Read the model definition and answer for the solid it produces. Units are mm, in the model's axes. A direction names the side the tool comes from. Round coordinates to 2 decimals unless told otherwise and drop trailing zeros. Write each loop counter-clockwise with the first axis right and the second up, starting at its lowest first coordinate (ties: lowest second). Pieces come first, ordered by that corner, then holes. Notation, with made-up numbers: (78.5, 85.25) - (118.5, 85.25) arc R16 cw to (118.5, 104.25) - close; hole circle Ø5 at (86, 26). An arc over 180 degrees is marked (long way). Use one line per item in the form item = value. Start each with the question number.
1) For a pull along Y with two mould halves and no side action, classify faces 1 (the face through (-12, -8, -5)), 2 (the face through (0, -2.8, 9.3)), 3 (the face through (-0.61, 13, 4.09)) as released by +Y, released by -Y, zero draft, split by the parting line, or undercut.
2) Consider line 1 along X through (y, z) = (16, -9.5); line 2 along Z through (x, y) = (-6.5, 12); line 3 along Z through (x, y) = (-7, -17.5). Determine where each line is inside the solid, lowest interval first. Write a range as from..to.
3) For faces 4 (the face through (-2, 13, -13)), 5 (the face through (-6.206, 4.57, 7.167)), 6 (the face through (-11.47, -1.46, 11.12)), determine the directions among +Z, -Z, +X, -X, +Y, -Y from which every point of the face is accessible in a straight line to the end or side of a thin tool.
4) The part is cut by section B-B, the plane x = -8. Give the vertices of the cut face in (y, z), plus the area to 3 significant figures.
5) The part is cut by section A-A, the plane x = -10.25. Give the vertices of the cut face in (y, z).
6) Each of these flat-tipped pins is pushed along its axis until it touches: pin 1 (3 mm diameter, centred on x = -8, y = 12.5, fed in from -Z); pin 2 (15.5 mm diameter, centred on y = 0, z = 0, fed in from -X); pin 3 (2 mm diameter, centred on x = -2, z = -3.5, fed in from -Y); pin 4 (6 mm diameter, centred on x = -10, z = -9, fed in from +Y). Where does it stop, or does it pass through?
from build123d import *


with BuildPart() as part:
    # OutRacSke → OuterRace (revolve)
    with BuildSketch(Plane.XY):
        with BuildLine():
            Line((-2, 18.15674466), (-13, 15.704))
            Line((-13, 15.704), (-13, 19))
            ThreePointArc((-13, 19), (-12.707106781, 19.707106781), (-12, 20))
            Line((-12, 20), (-2.44, 20))
            Line((-2.44, 20), (-2, 19.56))
            Line((-2, 19.56), (-2, 18.15674466))
        make_face()
    revolve(axis=Axis((-42.5, 0, 0), (1, 0, 0)))

    # RolSimSke → RollersSimplified (revolve)
    with BuildSketch(Plane.XY):
        Polygon((-12, 16.006611671), (-2.337294608, 18.161170676), (-1.211047855, 13.110211039), (-10.873753248, 10.955652034), align=None)
    revolve(axis=Axis((0, 0, 0), (-1, 0, 0)))

    # InsRacSke → InnerRace (revolve)
    with BuildSketch(Plane.XY):
        with BuildLine():
            Line((-10.925817259, 11.214402034), (-12, 11.214402034))
            Line((-12, 11.214402034), (-12, 8.94))
            Line((-12, 8.94), (-11.56, 8.5))
            Line((-11.56, 8.5), (-1, 8.5))
            ThreePointArc((-1, 8.5), (-0.292893219, 8.792893219), (0, 9.5))
            Line((0, 9.5), (0, 13.627711039))
            Line((0, 13.627711039), (-1.205416623, 13.627711039))
            Line((-1.205416623, 13.627711039), (-1.205416623, 13.110211039))
            Line((-1.205416623, 13.110211039), (-10.868122015, 10.955652034))
            Line((-10.868122015, 10.955652034), (-10.925817259, 11.214402034))
        make_face()
    revolve(axis=Axis((-42.5, 0, 0), (1, 0, 0)))


solid = part.part
Geometry results:
q1.face_1 = undercut
q1.face_2 = zero draft
q1.face_3 = split by the parting line
q2.line_1 = -13..-2
q2.line_2 = -16..16
q2.line_3 = -9.68..9.68
q3.face_4 = +X
q3.face_5 = +X, -X
q3.face_6 = -X
q4.outline = circle Ø40 at (0, 0); circle Ø23.19 at (0, 0); hole circle Ø23.19 at (0, 0); hole circle Ø17 at (0, 0)
q4.area = 1,030 mm2
q5.outline = circle Ø40 at (0, 0); circle Ø22.19 at (0, 0); hole circle Ø22.19 at (0, 0); hole circle Ø17 at (0, 0)
q6.pin_1 = -16.7
q6.pin_2 = through
q6.pin_3 = -19.83
q6.pin_4 = 19.08
